The model under review builds one solid part; all positions refer to its coordinate system, in mm. Round coordinates to 2 decimals unless told otherwise and drop trailing zeros. Order: outer loops, then holes, each group sorted by start corner. A loop starts at its lowest first (then second) coordinate and runs counter-clockwise, first axis right, second up. Notation, with made-up numbers: M 21,0.5 L 58,0.5 A13 ccw 58,10.5 Z; hole C 53,58 d7. An arc over 180 degrees is marked long. Answer as a JSON object with one key per item and string values. Group by question number.
1. Clearance check with flat-ended pins moving along their axes: P1, Ø10, axis at x = 201.5, y = -88.5, coming from the -Z side; P2, Ø10, axis at x = 416, z = 8, coming from the -Y side. State where each tip first meets the part, or that it passes through.
2. Add section C-C on y = -79. State the section outline as (x, z) points (3 decimals).
3. Add section A-A on x = 410.5. State the section outline as (y, z) points.
4. Add section B-B on z = 11. State the section outline as (x, y) points (3 decimals).
5. To check wall thickness, follow probe 1 along Y at (x, z) = (191, 17); probe 2 along Y at (x, z) = (442, 22); probe 3 along Z at (x, y) = (80, -75). State the ranges of each line that lie inside material, in increasing order. Write a range as [from, to].
Autodesk Inventor part; units mm, degrees
ref_plane "YZ Plane" through (0, 0, 0) normal (1, 0, 0) x (0, 1, 0)
ref_plane "XZ Plane" through (0, 0, 0) normal (0, 1, 0) x (-1, 0, 0)
ref_plane "XY Plane" through (0, 0, 0) normal (0, 0, 1) x (1, 0, 0)
sketch "Sketch1" plane through (0, 0, 0) normal (0, 0, 1) x (1, 0, 0)
  line L0 (0, 0) -> (-92.075, 0)
  line L1 (-92.075, 0) -> (-92.075, 25.4)
  line L2 (-92.075, 25.4) -> (-92.075, -101.6)
  line L3 (-92.075, -101.6) -> (492.125, -101.6)
  line L4 (492.125, -101.6) -> (492.125, 25.4)
  line L5 (492.125, 25.4) -> (-92.075, 25.4)
  dimension "d0" = 92.075
  dimension "d1" = 25.4
  dimension "d2" = 127
  dimension "d3" = 0
  dimension "d4" = 584.2
  dimension "d5" = 90
  dimension "d6" = 127
  dimension "d7" = 90
extrude "Extrusion1" add sketch "Sketch1" along normal blind 76.2
fillet "Fillet1" radius 31.75 2 edges at (200.025, 25.4, 0) (200.025, -101.6, 0)
properties part number "BumperFront"
Recorded:
{
 "1": {"P1": "stops at z = 3.08", "P2": "stops at y = -95.47"},
 "2": {"outline": "M -92.075,1.347 L 492.125,1.347 L 492.125,76.2 L -92.075,76.2 Z"},
 "3": {"outline": "M -101.6,31.75 A31.75 ccw -69.85,0 L -6.35,0 A31.75 ccw 25.4,31.75 L 25.4,76.2 L -101.6,76.2 Z"},
 "4": {"outline": "M -92.075,-93.881 L 492.125,-93.881 L 492.125,17.681 L -92.075,17.681 Z"},
 "5": {"probe 1": "y = [-97.97, 21.77]", "probe 2": "y = [-100.07, 23.87]", "probe 3": "z = [0.42, 76.2]"}
}
